```python
from build123d import *

# Parameters (mm, degrees)
F0_W     = 290
F0_H     = 238.5
F0_W_2   = 240
F0_H_2   = 188.5
F1_DEPTH = 50
F2_R     = 15
F3_DEPTH = 238.501
F4_R     = 5
F5_DEPTH = 290.001


with BuildPart() as f1:
    # F0 (on Front) → F1 (new body, symmetric)
    with BuildSketch(Plane.XZ):
        with Locations((0, -11.25)):
            Rectangle(F0_W, F0_H)
        with Locations((0, -11.25)):
            Rectangle(F0_W_2, F0_H_2, mode=Mode.SUBTRACT)
    extrude(amount=F1_DEPTH, both=True)

    # F2 (on face) → F3 (cut, through all)
    with BuildSketch(Plane.XY.offset(108)):
        with Locations((0, -20)):
            Circle(F2_R)
    extrude(amount=-F3_DEPTH, mode=Mode.SUBTRACT)

    # F4 (on face) → F5 (cut, through all)
    with BuildSketch(Plane.YZ.offset(145)):
        with Locations((10, 55)):
            Circle(F4_R)
        with Locations((10, -55)):
            Circle(F4_R)
    extrude(amount=-F5_DEPTH, mode=Mode.SUBTRACT)


solid = f1.part
```
Geometry check sheet. Reference: the model listing, model coordinates, mm. A direction names the side the tool comes from. Give positions to 0.01 mm unless a question says otherwise; leave off trailing zeros. Order: outer loops, then holes, each group sorted by start corner. A loop starts at its lowest first (then second) coordinate and runs counter-clockwise, first axis right, second up.
1. Access from +Z, -Z, +X, -X, +Y, -Y to the whole of each face (thin tool, end or side, straight path). Record for faces 4 (the face through (-132, 13, -51)), 5 (the face through (-2, -1, 83)).
2. Section check B-B, the plane z = -12.5. Enter the section's corners in (x, y), and give its area (3 significant figures).
3. Section check C-C, the plane x = -49.5. Enter the section's corners in (y, z), and give its area (3 significant figures).
4. Section check D-D, the plane z = -55. Enter the section's corners in (x, y), and give its area (3 significant figures).
5. Section check A-A, the plane y = -20. Enter the section's corners in (x, z).
6. Release check for a two-part mould opening along X. For faces 1 (the face through (-2, 50, -116)), 2 (the face through (145, -1, -13)), 3 (the face through (-120, -1, -13)) record: pulls with the +X half, pulls with the -X half, needs draft (parallel to the pull), parting line crosses it, or undercut.
7. Thickness scan on L1, parallel to Z at x = 139.5, y = 10; L2, parallel to X at y = 34.5, z = -67; L3, parallel to Z at x = -53, y = -0.5. Record the ranges inside material, lowest first.
Values follow:
1. face 4: +X, -X
1. face 5: +Y, -Y
2. outline: (-145, -50) - (-120, -50) - (-120, 50) - (-145, 50) - close; (120, -50) - (145, -50) - (145, 50) - (120, 50) - close
2. area: 5,000 mm2
3. outline: (-50, -130.5) - (50, -130.5) - (50, -105.5) - (-50, -105.5) - close; (-50, 83) - (50, 83) - (50, 108) - (-50, 108) - close
3. area: 5,000 mm2
4. outline: (-145, -50) - (-120, -50) - (-120, 5) - (-145, 5) - close; (-145, 15) - (-120, 15) - (-120, 50) - (-145, 50) - close; (120, -50) - (145, -50) - (145, 5) - (120, 5) - close; (120, 15) - (145, 15) - (145, 50) - (120, 50) - close
4. area: 4,500 mm2
5. outline: (-145, -130.5) - (-15, -130.5) - (-15, -105.5) - (-120, -105.5) - (-120, 83) - (-15, 83) - (-15, 108) - (-145, 108) - close; (15, -130.5) - (145, -130.5) - (145, 108) - (15, 108) - (15, 83) - (120, 83) - (120, -105.5) - (15, -105.5) - close
6. face 1: needs draft
6. face 2: pulls with the +X half
6. face 3: undercut
7. L1: z = -130.5 to -60, -50 to 50, 60 to 108
7. L2: x = -145 to -120, 120 to 145
7. L3: z = -130.5 to -105.5, 83 to 108
